Can you work these out from the model? Positions are in its coordinate system, mm. A direction names the side the tool comes from. Round coordinates to 2 decimals unless told otherwise and drop trailing zeros. Write each loop counter-clockwise with the first axis right and the second up, starting at its lowest first coordinate (ties: lowest second). Pieces come first, ordered by that corner, then holes. Notation, with made-up numbers: M 27.25,28 L 46.25,28 A29 cw 46.25,62 Z; hole C 54.5,-1.75 d8. An arc over 180 degrees is marked long. Use one line per item in the form item = value. Start each with the question number.
```python
from build123d import *

# Parameters (mm, degrees)
SKETCH1_W           = 75
SKETCH1_H           = 75
SKETCH1_R           = 2.5
SKETCH1_R_2         = 7.5
BOSS_EXTRUDE1_DEPTH = 6
SKETCH2_W           = 69
SKETCH2_H           = 69
CUT_EXTRUDE1_DEPTH  = 3
FILLET1_R           = 8


with BuildPart() as part:
    # Sketch1 → Boss-Extrude1 (new body)
    with BuildSketch(Plane.XY):
        with Locations((37.5, 37.5)):
            Rectangle(SKETCH1_W, SKETCH1_H)
        with Locations((7, 68)):
            Circle(SKETCH1_R, mode=Mode.SUBTRACT)
        with Locations(Location((68, 68, 0), (0, 0, 180))):
            Circle(SKETCH1_R, mode=Mode.SUBTRACT)
        with Locations((68, 7)):
            Circle(SKETCH1_R, mode=Mode.SUBTRACT)
        with Locations(Location((7, 7, 0), (0, 0, 180))):
            Circle(SKETCH1_R, mode=Mode.SUBTRACT)
        with Locations((37.5, 37.5)):
            Circle(SKETCH1_R_2, mode=Mode.SUBTRACT)
    extrude(amount=BOSS_EXTRUDE1_DEPTH)

    # Sketch2 → Cut-Extrude1 (cut)
    with BuildSketch(Plane.XY.offset(6)):
        with Locations((37.5, 37.5)):
            Rectangle(SKETCH2_W, SKETCH2_H)
    extrude(amount=-CUT_EXTRUDE1_DEPTH, mode=Mode.SUBTRACT)

    # Fillet1
    fillet1_edges = [part.edges().sort_by_distance(p)[0] for p in [
        (0, 75, 3),
        (75, 75, 3),
        (75, 0, 3),
        (0, 0, 3),
    ]]
    fillet(fillet1_edges, radius=FILLET1_R)


solid = part.part
```
1. If we mould it in two halves opening along Y, with no side actions, what happens to faces 1 (the face through (37, 29.7, 0)), 2 (the face through (8.15, 65.78, 1.48)), 3 (the face through (72.594, 2.281, 3.042)), 4 (the face through (35.87, 30.18, 1.48))? For each: pulls with the +Y half, pulls with the -Y half, needs draft (parallel to the pull), parting line crosses it, or undercut.
2. If we section it at B-B (y = 7): List the corners of the cut face in (x, z) for me.
3. Please list where these lines run through material, in increasing order: line 1 along X through (y, z) = (23, 3.2); line 2 along Y through (x, z) = (68, 0.85).
4. If we section it at A-A (z = 1.4): List the corners of the cut face in (x, y) for me, and give its area (3 significant figures).
5. Which directions (+Z, -Z, +X, -X, +Y, -Y) give clear straight access to the entire face, cutting with the end or side of a thin tool? Please do faces 5 (the face through (37, 3, 5)), 6 (the face through (75, 37, 3)).
6. If we section it at C-C (x = 40): List the corners of the cut face in (y, z) for me.
7. If we section it at D-D (y = 50): List the corners of the cut face in (x, z) for me, and give its area (3 significant figures).
8. Will this pin go through, and if not, where does the flat tip stop? pin 1 (4 mm diameter, centred on x = 30, y = 56, fed in from +Z).
Model answer:
q1.face_1 = needs draft
q1.face_2 = undercut
q1.face_3 = pulls with the -Y half
q1.face_4 = undercut
q2.outline = M 0.06,0 L 4.5,0 L 4.5,3 L 3,3 L 3,6 L 0.06,6 Z; M 9.5,0 L 65.5,0 L 65.5,3 L 9.5,3 Z; M 70.5,0 L 74.94,0 L 74.94,6 L 72,6 L 72,3 L 70.5,3 Z
q3.line_1 = 0 to 3, 72 to 75
q3.line_2 = 0.06 to 4.5, 9.5 to 65.5, 70.5 to 74.94
q4.outline = M 0,8 A8 ccw 8,0 L 67,0 A8 ccw 75,8 L 75,67 A8 ccw 67,75 L 8,75 A8 ccw 0,67 Z; hole C 7,7 d5; hole C 7,68 d5; hole C 37.5,37.5 d15; hole C 68,7 d5; hole C 68,68 d5
q4.area = 5,310 mm2
q5.face_5 = +Z
q5.face_6 = +Z, -Z, +X, +Y, -Y
q6.outline = M 0,0 L 30.43,0 L 30.43,3 L 3,3 L 3,6 L 0,6 Z; M 44.57,0 L 75,0 L 75,6 L 72,6 L 72,3 L 44.57,3 Z
q7.outline = M 0,0 L 75,0 L 75,6 L 72,6 L 72,3 L 3,3 L 3,6 L 0,6 Z
q7.area = 243 mm2
q8.pin_1 = 3
